Source: CAD feature listing. Evaluate the final solid. Frame: model axes, mm. Face numbers are marked on the shaded views. A direction names the side the tool comes from. Coordinates: 2 decimals unless noted, no trailing zeros. Write each loop counter-clockwise with the first axis right and the second up, starting at its lowest first coordinate (ties: lowest second). Pieces come first, ordered by that corner, then holes. Notation, with made-up numbers: M 45.25,-28 L 59.25,-28 A14 ccw 59.25,-11 Z; hole C -28.5,-14.75 d4. An arc over 180 degrees is marked long. Answer as CSV lines item,"result". Start each with the question number.
1. Section C-C on x = 1. Return the cut outline in (y, z).
2. Section A-A on x = -14. Return the cut outline in (y, z), plus the area to 4 significant figures.
3. Line query: probe 1 along Y at (x, z) = (-12, -2); probe 2 along Z at (x, y) = (-14, 16.8); probe 3 along X at (y, z) = (17.1, 0). Output: solid intervals per line, ascending. Write a range as [from, to].
4. Section D-D on z = 3.5. Return the cut outline in (x, y), plus the area to 3 significant figures.
5. Section B-B on x = 14. Return the cut outline in (y, z), plus the area to 4 significant figures.
6. Mould query, pull axis Y, two halves, no side actions, for the marked faces 4, 5 and 6. Classes: pulls with the +Y half, pulls with the -Y half, needs draft (parallel to the pull), parting line crosses it, or undercut.
7. Reachability of the marked faces 1, 2 and 3 from +Z, -Z, +X, -X, +Y, -Y: full face, straight path, thin tool, end or side. Return the list, or none.
8. Contact query for flat-ended pins moving along their axis: pin 1 Ø2 at (x, y) = (-12, 13) entering from -Z; pin 2 Ø1.5 at (x, z) = (-13.5, 0) entering from +Y; pin 3 Ø4 at (y, z) = (10.5, 0) entering from +X; pin 4 Ø2 at (x, y) = (-13, 5) entering from +Z. Output: stop coordinate, or through.
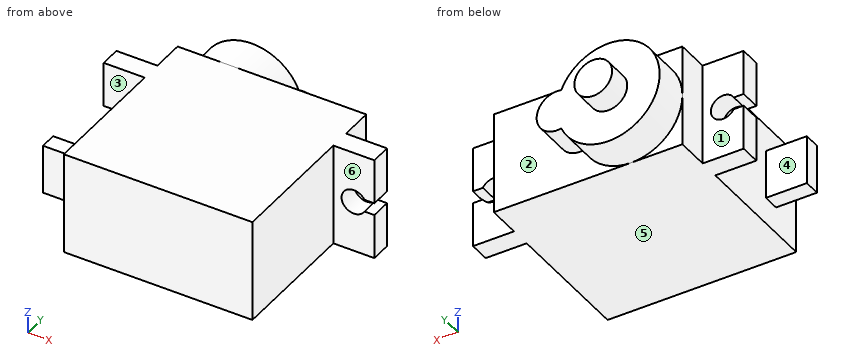
```python
from build123d import *

# Parameters (mm, degrees)
SKETCH1_W           = 23
SKETCH1_H           = 12.5
BOSS_EXTRUDE1_DEPTH = 22.5
BOSS_EXTRUDE2_DEPTH = 2.5
BOSS_EXTRUDE3_DEPTH = 4.5
SKETCH4_R           = 2.3
BOSS_EXTRUDE4_DEPTH = 3
SKETCH6_W           = 6
SKETCH6_H           = 2
BOSS_EXTRUDE6_DEPTH = 5


with BuildPart() as part:
    # Sketch1 → Boss-Extrude1 (new body)
    with BuildSketch(Plane(origin=(0, 0, 0), x_dir=(1, 0, 0), z_dir=(0, 1, 0))):
        Rectangle(SKETCH1_W, SKETCH1_H)
    extrude(amount=BOSS_EXTRUDE1_DEPTH)

    # Sketch2 → Boss-Extrude2 (add)
    with BuildSketch(Plane(origin=(0, 16, 0), x_dir=(1, 0, 0), z_dir=(0, 1, 0))):
        with BuildLine():
            Line((11.5, 6.25), (16.5, 6.25))
            Line((16.5, 6.25), (16.5, 0.75))
            Line((16.5, 0.75), (15.299038106, 0.75))
            ThreePointArc((15.299038106, 0.75), (12.5, 0), (15.299038106, -0.75))
            Line((15.299038106, -0.75), (16.5, -0.75))
            Line((16.5, -0.75), (16.5, -6.25))
            Line((16.5, -6.25), (11.5, -6.25))
            Line((11.5, -6.25), (11.5, 6.25))
        make_face()
        with BuildLine():
            Line((-11.5, 6.25), (-11.5, -6.25))
            Line((-11.5, -6.25), (-16.5, -6.25))
            Line((-16.5, -6.25), (-16.5, -0.75))
            Line((-16.5, -0.75), (-15.299038106, -0.75))
            ThreePointArc((-15.299038106, -0.75), (-12.5, 0), (-15.299038106, 0.75))
            Line((-15.299038106, 0.75), (-16.5, 0.75))
            Line((-16.5, 0.75), (-16.5, 6.25))
            Line((-16.5, 6.25), (-11.5, 6.25))
        make_face()
    extrude(amount=BOSS_EXTRUDE2_DEPTH)

    # Sketch3 → Boss-Extrude3 (add)
    with BuildSketch(Plane(origin=(0, 22.5, 0), x_dir=(1, 0, 0), z_dir=(0, 1, 0))):
        with BuildLine():
            ThreePointArc((0.5, 2.449489743), (-11.5, 0), (0.5, -2.449489743))
            ThreePointArc((0.5, -2.449489743), (3.5, 0), (0.5, 2.449489743))
        make_face()
    extrude(amount=BOSS_EXTRUDE3_DEPTH)

    # Sketch4 → Boss-Extrude4 (add)
    with BuildSketch(Plane(origin=(0, 27, 0), x_dir=(1, 0, 0), z_dir=(0, 1, 0))):
        with Locations(Location((-5.25, 0, 0), (0, 0, 270))):
            Circle(SKETCH4_R)
    extrude(amount=BOSS_EXTRUDE4_DEPTH)

    # Sketch6 → Boss-Extrude6 (add)
    with BuildSketch(Plane.ZY.offset(11.5)):
        with Locations((0, 5)):
            Rectangle(SKETCH6_W, SKETCH6_H)
    extrude(amount=BOSS_EXTRUDE6_DEPTH)


solid = part.part
```
Values:
1,outline,"M 0,-6.25 L 22.5,-6.25 L 22.5,-2.5 L 27,-2.5 L 27,2.5 L 22.5,2.5 L 22.5,6.25 L 0,6.25 Z"
2,outline,"M 4,-3 L 6,-3 L 6,3 L 4,3 Z; M 16,-6.25 L 18.5,-6.25 L 18.5,-1.5 L 16,-1.5 Z; M 16,1.5 L 18.5,1.5 L 18.5,6.25 L 16,6.25 Z"
2,area,"35.75 mm²"
3,probe 1,"[4, 6], [16, 18.5]"
3,probe 2,"[-6.25, -1.5], [1.5, 6.25]"
3,probe 3,"[-12.5, 12.5]"
4,outline,"M -16.5,16 L -11.5,16 L -11.5,0 L 11.5,0 L 11.5,16 L 16.5,16 L 16.5,18.5 L 11.5,18.5 L 11.5,22.5 L -0.07,22.5 L -0.07,27 L -10.43,27 L -10.43,22.5 L -11.5,22.5 L -11.5,18.5 L -16.5,18.5 Z"
4,area,"589 mm²"
5,outline,"M 16,-6.25 L 18.5,-6.25 L 18.5,-1.5 L 16,-1.5 Z; M 16,1.5 L 18.5,1.5 L 18.5,6.25 L 16,6.25 Z"
5,area,"23.75 mm²"
6,face 4,"undercut"
6,face 5,"needs draft"
6,face 6,"pulls with the -Y half"
7,face 1,"+Z, -Z, -X, +Y"
7,face 2,"+X, +Y"
7,face 3,"+Z, -Z, -X"
8,pin 1,"z = -6.25"
8,pin 2,"y = 6"
8,pin 3,"x = 11.5"
8,pin 4,"z = 3"
